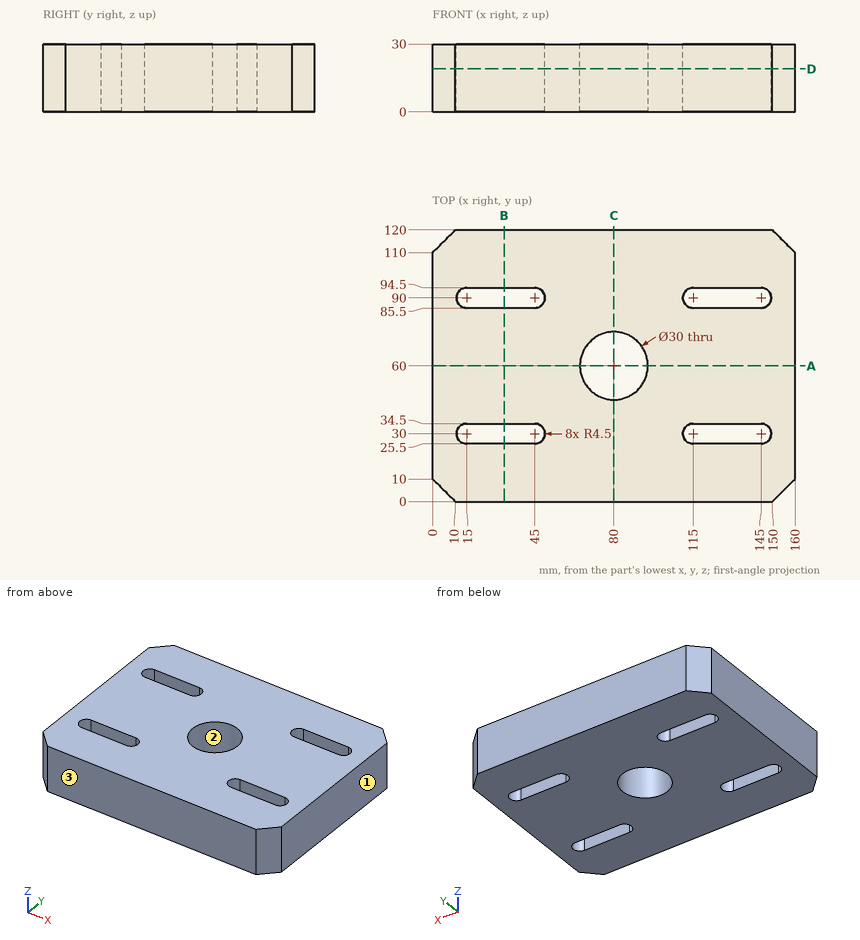
For this review, use the dimensioned drawing (mm, ordinates from the lowest corner) and the shaded views. Give positions to 0.01 mm unless a question says otherwise; leave off trailing zeros. Loops run counter-clockwise (first coordinate to the right, second up) from the corner with the lowest first, then second, coordinate; pieces in that order, holes last. Notation, with made-up numbers: (81, 25.25) -> (106, 25.25) arc R26 cw to (106, 44.25) -> close; hole circle Ø6 at (-10, -10.75). An arc over 180 degrees is marked (long way). One line per question, with ' | ' between items. Start each with the question number.
(1) We need section D-D (z = 19). State the section outline as (x, y) points.
(2) We need section C-C (x = 80). State the section outline as (y, z) points.
(3) For line 1 (Y direction, x = 119, z = 23.5); line 2 (Y direction, x = 80, z = 19); line 3 (X direction, y = 91.5, z = 6.5), list the stretches that pass through material, from the lowest coordinate up.
(4) Draft analysis for pull direction Y (two halves, no side actions). For the marked faces 1, 2 and 3, state which applies: +Y half, -Y half, draft (parallel to the pull), parting line (faces both ways), or undercut.
(5) We need section B-B (x = 31.5). State the section outline as (y, z) points.
(6) We need section A-A (y = 60). State the section outline as (x, z) points, and give its area (3 significant figures).
(7) Insertion check: P1, Ø24, axis at x = 80, y = 60, coming from the -Z side. The pin has a flat end and moves straight along its axis. Give the tip position at first contact, or say it passes through.
The answers:
1) outline: (0, 10) -> (10, 0) -> (150, 0) -> (160, 10) -> (160, 110) -> (150, 120) -> (10, 120) -> (0, 110) -> close; hole (15, 25.5) -> (45, 25.5) arc R4.5 ccw to (45, 34.5) -> (15, 34.5) arc R4.5 ccw to start; hole (15, 85.5) -> (45, 85.5) arc R4.5 ccw to (45, 94.5) -> (15, 94.5) arc R4.5 ccw to start; hole circle Ø30 at (80, 60); hole (115, 25.5) -> (145, 25.5) arc R4.5 ccw to (145, 34.5) -> (115, 34.5) arc R4.5 ccw to start; hole (115, 85.5) -> (145, 85.5) arc R4.5 ccw to (145, 94.5) -> (115, 94.5) arc R4.5 ccw to start
2) outline: (0, 0) -> (45, 0) -> (45, 30) -> (0, 30) -> close; (75, 0) -> (120, 0) -> (120, 30) -> (75, 30) -> close
3) line 1: y = 0 to 25.5, 34.5 to 85.5, 94.5 to 120 | line 2: y = 0 to 45, 75 to 120 | line 3: x = 0 to 10.76, 49.24 to 110.76, 149.24 to 160
4) face 1: draft | face 2: undercut | face 3: -Y half
5) outline: (0, 0) -> (25.5, 0) -> (25.5, 30) -> (0, 30) -> close; (34.5, 0) -> (85.5, 0) -> (85.5, 30) -> (34.5, 30) -> close; (94.5, 0) -> (120, 0) -> (120, 30) -> (94.5, 30) -> close
6) outline: (0, 0) -> (65, 0) -> (65, 30) -> (0, 30) -> close; (95, 0) -> (160, 0) -> (160, 30) -> (95, 30) -> close | area: 3,900 mm^2
7) P1: passes through
